Work out the finished part from the listing and answer in its coordinate system (mm). Face numbers are marked on the shaded views. A direction names the side the tool comes from. Coordinates: 2 decimals unless noted, no trailing zeros. Loops run counter-clockwise (first coordinate to the right, second up) from the corner with the lowest first, then second, coordinate; pieces in that order, holes last. Notation, with made-up numbers: (15, 44) - (30, 44) arc R25 ccw to (30, 74) - close; hole circle Ø3 at (59.5, -19). An arc over 180 degrees is marked (long way). Write each question's results on one line, items separated by ' | '. Start each with the question number.
Item 1: Section D-D, the plane y = 14 is taken. Write down the section's boundary in (x, z), plus the area to 3 significant figures.
Item 2: Consider probe 1 along Y at (x, z) = (2.1, 32); probe 2 along Y at (x, z) = (1.75, 9); probe 3 along Z at (x, y) = (37.5, 10). Determine where each line is inside the solid, lowest interval first. Write a range as [from, to].
Item 3: Section C-C, the plane z = 17.5 is taken. Write down the section's boundary in (x, y), plus the area to 3 significant figures.
Item 4: Section B-B, the plane x = 41 is taken. Write down the section's boundary in (y, z), plus the area to 3 significant figures.
Item 5: Section A-A, the plane y = 9 is taken. Write down the section's boundary in (x, z), plus the area to 3 significant figures.
Item 6: A tool of negligible diameter and unlimited length cuts with its end or side. For the marked faces 1 and 2, from which of +Z, -Z, +X, -X, +Y, -Y can it reach the whole face along a straight path? Write none if from no direction.
Item 7: Each of these flat-tipped pins is pushed along its axis until it touches: pin 1 Ø12 at (y, z) = (19.5, 11.5) entering from -X; pin 2 Ø5 at (y, z) = (25.5, 17.5) entering from +X; pin 3 Ø12 at (x, y) = (11.5, 21.5) entering from -Z. Where does it stop, or does it pass through?
from build123d import *

# Parameters (mm, degrees)
EXTRUDE_2_DEPTH     = 38
SKETCH_4_R          = 1.5
CUT_EXTRUDE_1_DEPTH = 50
SKETCH_5_R          = 1.5
CUT_EXTRUDE_2_DEPTH = 50


with BuildPart() as part:
    # 草图3 → 凸台-拉伸2 (new body)
    with BuildSketch(Plane(origin=(0, 0, 0), x_dir=(1, 0, 0), z_dir=(0, 1, 0))):
        Polygon((0, 0), (0, -50), (50, -50), (50, -47), (3, -47), (3, 0), align=None)
    extrude(amount=EXTRUDE_2_DEPTH)

    # 草图4 → 切除-拉伸1 (cut)
    with BuildSketch(Plane(origin=(3, 0, 0), x_dir=(0, 0, -1), z_dir=(1, 0, 0))):
        with Locations((-32, 29)):
            Circle(SKETCH_4_R)
        with Locations((-32, 9)):
            Circle(SKETCH_4_R)
        with Locations((-9, 19)):
            Circle(SKETCH_4_R)
    extrude(amount=-CUT_EXTRUDE_1_DEPTH, mode=Mode.SUBTRACT)

    # 草图5 → 切除-拉伸2 (cut)
    with BuildSketch(Plane(origin=(0, 0, 47), x_dir=(-1, 0, 0), z_dir=(0, 0, -1))):
        with Locations((-18, 29)):
            Circle(SKETCH_5_R)
        with Locations((-18, 9)):
            Circle(SKETCH_5_R)
        with Locations((-41, 19)):
            Circle(SKETCH_5_R)
    extrude(amount=-CUT_EXTRUDE_2_DEPTH, mode=Mode.SUBTRACT)


solid = part.part
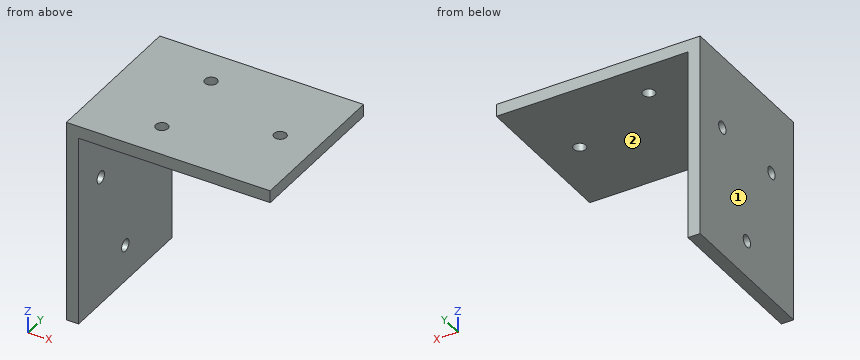
Answer key:
1) outline: (0, 0) - (3, 0) - (3, 47) - (50, 47) - (50, 50) - (0, 50) - close | area: 291 mm^2
2) probe 1: y = [0, 7.5], [10.5, 27.5], [30.5, 38] | probe 2: y = [0, 17.5], [20.5, 38] | probe 3: z = [47, 50]
3) outline: (0, 0) - (3, 0) - (3, 38) - (0, 38) - close | area: 114 mm^2
4) outline: (0, 47) - (17.5, 47) - (17.5, 50) - (0, 50) - close; (20.5, 47) - (38, 47) - (38, 50) - (20.5, 50) - close | area: 105 mm^2
5) outline: (0, 0) - (3, 0) - (3, 30.5) - (0, 30.5) - close; (0, 33.5) - (3, 33.5) - (3, 47) - (16.5, 47) - (16.5, 50) - (0, 50) - close; (19.5, 47) - (50, 47) - (50, 50) - (19.5, 50) - close | area: 273 mm^2
6) face 1: +Z, -Z, -X, +Y, -Y | face 2: -Z, +X, +Y, -Y
7) pin 1: stops at x = 0 | pin 2: stops at x = 3 | pin 3: stops at z = 47
